```python
from build123d import *

# Parameters (mm, degrees)
F0_R     = 13.716
F1_DEPTH = 25.4
F3_R     = 1.5875
F2_R     = 1.5875
F4_DEPTH = 25.4


with BuildPart() as f1:
    # F0 (on Front) → F1 (new body)
    with BuildSketch(Plane.XZ):
        with BuildLine():
            Line((5.715, -29.7924076074), (5.715, -18.172541787))
            ThreePointArc((5.715, -18.172541787), (0, 18.9799369156), (-5.715, -18.172541787))
            Line((-5.715, -18.172541787), (-5.715, -29.7924076074))
            Line((-5.715, -29.7924076074), (-22.225, -29.5853535962))
            Line((-22.225, -29.5853535962), (-22.225, -39.7453535962))
            Line((-22.225, -39.7453535962), (22.225, -39.7453535962))
            Line((22.225, -39.7453535962), (22.225, -29.5853535962))
            Line((22.225, -29.5853535962), (5.715, -29.7924076074))
        make_face()
        Circle(F0_R, mode=Mode.SUBTRACT)
    extrude(amount=F1_DEPTH)

    # F3 (on face) + F2 (on face) → F4 (cut)
    with BuildSketch(Plane(origin=(-0.3744703333, 0, -29.8593838697), x_dir=(0.9999213693, 0, -0.0125401412), z_dir=(0.0125401412, 0, 0.9999213693))):
        with Locations((-13.5965987763, -12.7)):
            Circle(F3_R)
    with BuildSketch(Plane(origin=(0.3744703333, 0, -29.8593838697), x_dir=(0.9999213693, 0, 0.0125401412), z_dir=(-0.0125401412, 0, 0.9999213693))):
        with Locations((13.5965987763, -12.7)):
            Circle(F2_R)
    extrude(amount=-F4_DEPTH, dir=(0.0125401412, 0, 0.9999213693), mode=Mode.SUBTRACT)


solid = f1.part
```
Input: part model. Units: mm. Frame: model coordinates. A direction names the side the tool comes from. Coordinates: 2 decimals unless noted, no trailing zeros. Write each loop counter-clockwise with the first axis right and the second up, starting at its lowest first coordinate (ties: lowest second). Pieces come first, ordered by that corner, then holes. Notation, with made-up numbers: (-21.75, 11.5) -> (2.25, 11.5) arc R27 ccw to (2.25, 41.5) -> close; hole circle Ø1 at (27.25, -11). An arc over 180 degrees is marked (long way). Answer as a JSON object with one key per item and string values.
1. Section D-D on z = 4.5. Return the cut outline in (x, y).
Result set:
{"outline": "(-18.47, -25.4) -> (-12.96, -25.4) -> (-12.96, 0) -> (-18.47, 0) -> close; (12.96, -25.4) -> (18.47, -25.4) -> (18.47, 0) -> (12.96, 0) -> close"}
2. Access query for faces 4 (the face through (0.755, -12.522, 18.965)), 5 (the face through (-14.239, -11.126, -34.654)). Directions: +Z, -Z, +X, -X, +Y, -Y. A direction counts if a zero-diameter tool reaches every point of the face in a straight line with its end or side. Return the directions, or none.
Result set:
{"face 4": "+Y, -Y", "face 5": "none"}
3. First-contact query: P1, Ø1, axis at x = 10, z = -16.5, coming from the -Y side; P2, Ø6, axis at y = -19, z = -17.5, coming from the -X side; P3, Ø12, axis at y = -11, z = -19, coming from the -X side; P4, Ø3.5, axis at y = -9, z = -24, coming from the +X side (3 decimals). Flat tips, straight axial feed; report the tip coordinate or a pass-through.
Result set:
{"P1": "stops at y = -25.4", "P2": "stops at x = -12.34", "P3": "stops at x = -13.91", "P4": "stops at x = 5.715"}
4. Material intervals for line 1 (Z direction, x = -7, y = -15.5); line 2 (Z direction, x = 0, y = -18.5); line 3 (Z direction, x = 10, y = -5.25), sorted ascending. Write a range as from..to.
Result set:
{"line 1": "z = -39.75..-29.78, -17.72..-11.8, 11.8..17.64", "line 2": "z = -39.75..-13.72, 13.72..18.98", "line 3": "z = -39.75..-29.74, -16.21..-9.39, 9.39..16.14"}
5. Section B-B on y = -6.25. Return the cut outline in (x, z) (3 decimals), then the cut area to 3 significant figures.
Result set:
{"outline": "(-22.225, -39.745) -> (22.225, -39.745) -> (22.225, -29.585) -> (5.715, -29.792) -> (5.715, -18.173) arc R19.016 ccw (long way) to (-5.715, -18.173) -> (-5.715, -29.792) -> (-22.225, -29.585) -> close; hole circle Ø27.432 at (0, 0)", "area": "1,120 mm2"}
6. Section A-A on x = 0. Return the cut outline in (y, z), then the cut area to 3 significant figures.
Result set:
{"outline": "(-25.4, -39.75) -> (0, -39.75) -> (0, -13.72) -> (-25.4, -13.72) -> close; (-25.4, 13.72) -> (0, 13.72) -> (0, 18.98) -> (-25.4, 18.98) -> close", "area": "795 mm2"}
7. Mould query, pull axis Z, two halves, no side actions, for faces 1 (the face through (22.225, -13, -35)), 2 (the face through (0, -13, -39.745)), 3 (the face through (5.715, -13, -24)). Classes: released by +Z, released by -Z, zero draft, split by the parting line, or undercut.
Result set:
{"face 1": "zero draft", "face 2": "released by -Z", "face 3": "undercut"}
8. Section C-C on x = 10.5. Return the cut outline in (y, z), then the cut area to 3 significant figures.
Result set:
{"outline": "(-25.4, -39.75) -> (0, -39.75) -> (0, -29.73) -> (-25.4, -29.73) -> close; (-25.4, -15.89) -> (0, -15.89) -> (0, -8.82) -> (-25.4, -8.82) -> close; (-25.4, 8.82) -> (0, 8.82) -> (0, 15.82) -> (-25.4, 15.82) -> close", "area": "611 mm2"}
